Build history of the part. All positions in model axes, mm. A direction names the side the tool comes from. Give positions to 0.01 mm unless a question says otherwise; leave off trailing zeros. Loops run counter-clockwise (first coordinate to the right, second up) from the corner with the lowest first, then second, coordinate; pieces in that order, holes last.
1) 3-axis set-ups, long thin cutter, end or side, ignore diameter. For faces 1 (the flat face through (8, 34, 2.54)), 2 (the flat face through (9, 34, 0)): which of +Z, -Z, +X, -X, +Y, -Y reach the whole face in a straight line?
2) Band-saw the part on B-B on x = 10.5. List the corners of the cut face in (y, z).
3) Wall check: line 1 (Z direction, x = 4.5, y = 17); line 2 (X direction, y = 65.5, z = -16.5); line 3 (Y direction, x = 5.5, z = -6.5). Give the ranges that are in metal, low to high.
4) Flat gauge pins, fed straight in: P1, Ø8, axis at x = 2.5, z = -19.5, coming from the +Y side; P2, Ø3, axis at x = 6.5, z = -6, coming from the +Y side. Where does each tip first touch, or does it go through?
5) Band-saw the part on C-C on z = -10.5. List the corners of the cut face in (x, y), then the cut area to 3 significant figures.
6) Band-saw the part on A-A on y = 16. List the corners of the cut face in (x, z).
7) Band-saw the part on D-D on x = 19.5. List the corners of the cut face in (y, z), then the cut area to 3 significant figures.
8) Two-plate mould, pull along X, no slides. Class faces 3 (the flat face through (20.084, 33.904, -40.622)), 4 (the flat face through (9, 0, -19)), 5 (the flat face through (9, -2.54, -19)): +X half, -X half, draft (parallel to the pull), parting line (faces both ways), or undercut.
```python
from build123d import *

# Parameters (mm, degrees)
SKETCH1_W           = 23.876
SKETCH1_H           = 44.45
SKETCH1_W_2         = 18.796
SKETCH1_H_2         = 39.37
BOSS_EXTRUDE1_DEPTH = 69.342
SKETCH2_W           = 23.876
SKETCH2_H           = 44.45
BOSS_EXTRUDE2_DEPTH = 2.54
CHAMFER1_SIZE       = 2.54


with BuildPart() as part:
    # Sketch1 → Boss-Extrude1 (new body)
    with BuildSketch(Plane(origin=(0, 0, 0), x_dir=(1, 0, 0), z_dir=(0, 1, 0))):
        with Locations((9.398, 19.685)):
            Rectangle(SKETCH1_W, SKETCH1_H)
        with Locations((9.398, 19.685)):
            Rectangle(SKETCH1_W_2, SKETCH1_H_2, mode=Mode.SUBTRACT)
    extrude(amount=BOSS_EXTRUDE1_DEPTH)

    # Sketch2 → Boss-Extrude2 (add)
    with BuildSketch(Plane.XZ):
        with Locations((9.398, -19.685)):
            Rectangle(SKETCH2_W, SKETCH2_H)
    extrude(amount=BOSS_EXTRUDE2_DEPTH)

    # Chamfer1
    chamfer1_edges = [part.edges().sort_by_distance(p)[0] for p in [
        (21.336, 33.401, -41.91),
        (21.336, 33.401, 2.54),
    ]]
    chamfer(chamfer1_edges, length=CHAMFER1_SIZE)


solid = part.part
```
Findings below:
1. face 1: +Z, +X, -X, +Y, -Y
1. face 2: +Y
2. outline: (-2.54, -41.91) - (69.34, -41.91) - (69.34, -39.37) - (0, -39.37) - (0, 0) - (69.34, 0) - (69.34, 2.54) - (-2.54, 2.54) - close
3. line 1: z = -41.91 to -39.37, 0 to 2.54
3. line 2: x = -2.54 to 0, 18.8 to 21.34
3. line 3: y = -2.54 to 0
4. P1: stops at y = 69.34
4. P2: stops at y = 0
5. outline: (-2.54, -2.54) - (21.34, -2.54) - (21.34, 69.34) - (18.8, 69.34) - (18.8, 0) - (0, 0) - (0, 69.34) - (-2.54, 69.34) - close
5. area: 413 mm2
6. outline: (-2.54, -41.91) - (18.8, -41.91) - (21.34, -39.37) - (21.34, 0) - (18.8, 2.54) - (-2.54, 2.54) - close; hole (0, -39.37) - (18.8, -39.37) - (18.8, 0) - (0, 0) - close
7. outline: (-2.54, -41.21) - (69.34, -41.21) - (69.34, 1.84) - (-2.54, 1.84) - close
7. area: 3,090 mm2
8. face 3: +X half
8. face 4: undercut
8. face 5: draft
